Source: CAD feature listing. Evaluate the final solid. Frame: model axes, mm. A direction names the side the tool comes from. Coordinates: 2 decimals unless noted, no trailing zeros. Order: outer loops, then holes, each group sorted by start corner. A loop starts at its lowest first (then second) coordinate and runs counter-clockwise, first axis right, second up.
Item 1: Section D-D on z = 10. State how many separate pieces and enclosed holes the cut face has, then the cut area to 3 significant figures.
Item 2: Mould query, pull axis Y, two halves, no side actions, for faces 1 (the cylindrical face through (101.83, 58.57, 9.54)), 2 (the cylindrical face through (198.1, 19.48, 10.03)), 3 (the flat face through (104, 0, 6)), 4 (the flat face through (104, 87, 6)). Classes: released by +Y, released by -Y, zero draft, split by the parting line, or undercut.
Item 3: Section A-A on x = 122.5. Return the cut outline in (y, z) (3 decimals), then the cut area to 3 significant figures.
Item 4: Contact query for flat-ended pins moving along their axis: P1, Ø4, axis at x = 195, y = 18.5, coming from the +Z side; P2, Ø6, axis at x = 194, y = 18, coming from the -Z side. Output: stop coordinate, or through.
Item 5: Section B-B on y = 68.5. Return the cut outline in (x, z).
Item 6: Ray query, line 1 (Y direction, x = 15, z = 9.8); line 2 (Y direction, x = 195, z = 4); line 3 (Y direction, x = 105, z = 3). Return the intervals inside material, ascending.
Item 7: Section C-C on x = 15. Return the cut outline in (y, z), then the cut area to 3 significant figures.
Item 8: Reachability of faces 5 (the flat face through (18, 71, 8)), 6 (the flat face through (106, 29, 7)), 7 (the cylindrical face through (125.36, 44.4, 3.55)) from +Z, -Z, +X, -X, +Y, -Y: full face, straight path, thin tool, end or side. Return the list, or none.
from build123d import *

# Parameters (mm, degrees)
F0_W      = 210
F0_H      = 87
F1_DEPTH  = 12
F2_R      = 3.25
F3_DEPTH  = 12.001
F4_R      = 13.5
F5_DEPTH  = 12.001
F6_R      = 3
F7_DEPTH  = 12.001
F8_R      = 3.995
F9_DEPTH  = 5
F10_R     = 6
F11_DEPTH = 8


with BuildPart() as f1:
    # F0 (on Top) → F1 (new body)
    with BuildSketch(Plane.XY):
        with Locations((105, 43.5)):
            Rectangle(F0_W, F0_H)
    extrude(amount=F1_DEPTH)

    # F2 (on face) → F3 (cut, through all)
    with BuildSketch(Plane.XY.offset(12)):
        with Locations((15, 68.5)):
            Circle(F2_R)
        with Locations((195, 68.5)):
            Circle(F2_R)
        with Locations((195, 18.5)):
            Circle(F2_R)
        with Locations((15, 18.5)):
            Circle(F2_R)
    extrude(amount=-F3_DEPTH, mode=Mode.SUBTRACT)

    # F4 (on face) → F5 (cut, through all)
    with BuildSketch(Plane.XY.offset(12)):
        with Locations((105, 43.5)):
            Circle(F4_R)
    extrude(amount=-F5_DEPTH, mode=Mode.SUBTRACT)

    # F6 (on face) → F7 (cut, through all)
    with BuildSketch(Plane.XY.offset(12)):
        with Locations((105, 61)):
            Circle(F6_R)
        with Locations((87.5, 43.5)):
            Circle(F6_R)
        with Locations((105, 26)):
            Circle(F6_R)
        with Locations((122.5, 43.5)):
            Circle(F6_R)
    extrude(amount=-F7_DEPTH, mode=Mode.SUBTRACT)

    # F8 (on face) → F9 (cut)
    with BuildSketch(Plane.XY.offset(12)):
        with Locations((105, 61)):
            Circle(F8_R)
        with Locations((87.5, 43.5)):
            Circle(F8_R)
        with Locations((105, 26)):
            Circle(F8_R)
        with Locations((122.5, 43.5)):
            Circle(F8_R)
    extrude(amount=-F9_DEPTH, mode=Mode.SUBTRACT)

    # F10 (on face) → F11 (cut)
    with BuildSketch(Plane(origin=(0, 0, 0), x_dir=(1, 0, 0), z_dir=(0, 0, -1))):
        with Locations((15, -18.5)):
            Circle(F10_R)
        with Locations((15, -68.5)):
            Circle(F10_R)
        with Locations((195, -18.5)):
            Circle(F10_R)
        with Locations((195, -68.5)):
            Circle(F10_R)
    extrude(amount=-F11_DEPTH, mode=Mode.SUBTRACT)


solid = f1.part
Answer list:
1. separate pieces: 1
1. enclosed holes: 9
1. area: 17,400 mm2
2. face 1: undercut
2. face 2: undercut
2. face 3: released by -Y
2. face 4: released by +Y
3. outline: (0, 0) - (40.5, 0) - (40.5, 7) - (39.505, 7) - (39.505, 12) - (0, 12) - close; (46.5, 0) - (87, 0) - (87, 12) - (47.495, 12) - (47.495, 7) - (46.5, 7) - close
3. area: 962 mm2
4. P1: passes through
4. P2: stops at z = 8
5. outline: (0, 0) - (9, 0) - (9, 8) - (11.75, 8) - (11.75, 12) - (0, 12) - close; (18.25, 8) - (21, 8) - (21, 0) - (189, 0) - (189, 8) - (191.75, 8) - (191.75, 12) - (18.25, 12) - close; (198.25, 8) - (201, 8) - (201, 0) - (210, 0) - (210, 12) - (198.25, 12) - close
6. line 1: y = 0 to 15.25, 21.75 to 65.25, 71.75 to 87
6. line 2: y = 0 to 12.5, 24.5 to 62.5, 74.5 to 87
6. line 3: y = 0 to 23, 29 to 30, 57 to 58, 64 to 87
7. outline: (0, 0) - (12.5, 0) - (12.5, 8) - (15.25, 8) - (15.25, 12) - (0, 12) - close; (21.75, 8) - (24.5, 8) - (24.5, 0) - (62.5, 0) - (62.5, 8) - (65.25, 8) - (65.25, 12) - (21.75, 12) - close; (71.75, 8) - (74.5, 8) - (74.5, 0) - (87, 0) - (87, 12) - (71.75, 12) - close
7. area: 800 mm2
8. face 5: -Z
8. face 6: +Z
8. face 7: +Z, -Z
